Autodesk Fusion 360 part; units mm, degrees
sketch "Sketch1" plane through (0, 0, 0) normal (0, 0, 1) x (1, 0, 0)
  line L0 (0, 0) -> (28, 0)
  line L1 (28, 0) -> (28, 16)
  line L2 (28, 16) -> (0, 16)
  line L3 (0, 16) -> (0, 0)
  dimension "d1" = 28
  dimension "d2" = 16
extrude "Extrude1" add sketch "Sketch1" along normal blind 16
sketch "Sketch2" plane through (0, 0, 16) normal (0, 0, 1) x (-1, 0, 0)
  line L0 (0, -16) -> (0, 0)
  line L1 (0, 0) -> (-28, 0)
  line L2 (-28, 0) -> (-28, -16)
  line L3 (-28, -16) -> (0, -16)
  line L4 (0, -8) -> (-28, -8) construction
  line L5 (-6.5, -16) -> (-6.5, 0) construction
  line L6 (-22, -16) -> (-22, 0) construction
  circle A0 centre (-6.5, -8) radius 3.25
  circle A1 centre (-22, -8) radius 3.25
  dimension "d5" = 6.5
  dimension "d6" = 15.5
  dimension "d7" = 6.5
  dimension "d8" = 6.5
extrude "Extrude2" cut sketch "Sketch2" against normal blind 6 contours A0 | A1
sketch "Sketch3" plane through (0, 0, 0) normal (0, 0, -1) x (1, 0, 0)
  line L0 (0, 0) -> (0, -16)
  line L1 (0, -16) -> (28, -16)
  line L2 (28, -16) -> (28, 0)
  line L3 (28, 0) -> (0, 0)
  circle A0 centre (6.5, -8) radius 3.25
  circle A1 centre (22, -8) radius 3.25
extrude "Extrude3" cut sketch "Sketch3" against normal blind 6 contours A0 | A1
sketch "Sketch4" plane through (28, 0, 0) normal (1, 0, 0) x (0, 1, 0)
  line L0 (0, 0) -> (16, 0)
  line L1 (16, 0) -> (16, 16)
  line L2 (16, 16) -> (0, 16)
  line L3 (0, 16) -> (0, 0)
  line L4 (7.6128, 11.7945) -> (5.4221, 8)
  line L5 (12.2966, 8) -> (10.1058, 4.2055)
  line L6 (2.0465, 11.4373) -> (8, 14.8745)
  line L7 (5.8942, 11.7945) -> (7.6128, 11.7945)
  line L8 (3.7034, 8) -> (5.8942, 11.7945)
  line L9 (9.3314, 11.7945) -> (4.95, 4.2055)
  line L10 (13.9535, 11.4373) -> (13.9535, 4.5627)
  line L11 (6.6686, 4.2055) -> (11.05, 11.7945)
  line L12 (10.5779, 8) -> (12.2966, 8)
  line L13 (8, 14.8745) -> (13.9535, 11.4373)
  line L14 (8, 1.1255) -> (2.0465, 4.5627)
  line L15 (2.0465, 4.5627) -> (2.0465, 11.4373)
  line L16 (8.3872, 4.2055) -> (10.5779, 8)
  line L17 (5.4221, 8) -> (3.7034, 8)
  line L18 (4.95, 4.2055) -> (6.6686, 4.2055)
  line L19 (11.05, 11.7945) -> (9.3314, 11.7945)
  line L20 (10.1058, 4.2055) -> (8.3872, 4.2055)
  line L21 (13.9535, 4.5627) -> (8, 1.1255)
  line L22 (7.0257, 8) -> (8.9743, 8) construction
  line L23 (0, 8) -> (16, 8) construction
  line L24 (8, 16) -> (8, 0) construction
  point P0 (8, 8)
  point P1 (8, 8)
extrude "Extrude4" add sketch "Sketch4" along normal blind 0.4 contours L6 L10 L13 L14 L15 L21
sketch "Sketch5" plane through (0, 0, 0) normal (0, -1, 0) x (1, 0, 0)
  line L0 (0, 0) -> (28, 0)
  line L1 (28, 0) -> (28, 16)
  line L2 (28, 16) -> (0, 16)
  line L3 (0, 16) -> (0, 0)
  arc A0 (28, 9.8) -> (28, 6.2) centre (28, 8) ccw
  dimension "d25" = 1.8
sketch "Sketch6" plane through (0, 16, 0) normal (0, 1, 0) x (-1, 0, 0)
  line L0 (-28, 0) -> (0, 0)
  line L1 (0, 0) -> (0, 16)
  line L2 (0, 16) -> (-28, 16)
  line L3 (-28, 16) -> (-28, 0)
  arc A0 (-28, 6.2) -> (-28, 9.8) centre (-28, 8) ccw
extrude "Extrude8" cut sketch "Sketch5" against normal blind 2.0465 contours L1 A0
extrude "Extrude9" cut sketch "Sketch6" against normal blind 2.047 contours L3 A0
chamfer "Chamfer1" distance 0.4 angle 45 20 edges at (14, 0, 16) (28, 8, 16) (28, 0, 3.1) (28, 0, 12.9) (28, 16, 3.1) (28, 16, 12.9) (14, 16, 16) (0, 8, 16) (0, 16, 8) (14, 16, 0) (14, 0, 0) (0, 8, 0) (0, 0, 8) (28, 8, 0) (26.2, 0, 8) (28, 1.0232, 6.2) (28, 1.0232, 9.8) (26.2, 16, 8) (28, 14.9768, 6.2) (28, 14.9768, 9.8)
chamfer "Chamfer2" distance 0.4 angle 45 6 edges at (28.4, 5.0233, 13.1559) (28.4, 10.9768, 13.1559) (28.4, 2.0465, 8) (28.4, 5.0232, 2.8441) (28.4, 10.9768, 2.8441) (28.4, 13.9535, 8)
chamfer "Chamfer3" distance 0.4 angle 45 4 edges at (9.5301, 6.8247, 16) (25.0301, 6.8247, 16) (3.4699, 6.8247, 0) (18.9699, 6.8247, 0)
chamfer "Chamfer4" distance 0.6 angle 45 4 edges at (25.0301, 6.8247, 10) (9.5301, 6.8247, 10) (18.9699, 6.8247, 6) (3.4699, 6.8247, 6)
extrude "Extrude7" cut 2 faces at (7.0507, 8.6906, 10) (23.3948, 7.2286, 10) along direction (0, 0, -1) blind 4
For this review, take the finished solid that the model builds, in its own axes (mm). A direction names the side the tool comes from. Round coordinates to 2 decimals unless told otherwise and drop trailing zeros. Write each loop counter-clockwise with the first axis right and the second up, starting at its lowest first coordinate (ties: lowest second). Pieces come first, ordered by that corner, then holes. Notation, with made-up numbers: (-19, -3) -> (40, -3) arc R23 ccw to (40, 28) -> close; hole circle Ø10 at (-38.75, 34). An arc over 180 degrees is marked (long way). Put each result on its own line as item: value.
Q1. Machinability: for faces 4 (the cylindrical face through (25.247, 7.857, 13.135)), 5 (the cylindrical face through (20.777, 10.351, 8.028)), 6 (the flat face through (28, 10, 6)), which of the approach directions +Z, -Z, +X, -X, +Y, -Y give a long, thin tool a straight path to every point of the face, cutting with its end or side? Answer none if there is none.
Determined:
face 4: +Z
face 5: +Z, -Z
face 6: +X
Q2. To check wall thickness, follow L1, parallel to X at y = 8, z = 13.3; L2, parallel to X at y = 8, z = 9.15; L3, parallel to Y at x = 6, z = 13.25. State the ranges of each line that lie inside material, in increasing order. Write a range as [from, to].
Determined:
L1: x = [0, 3.25], [9.75, 18.75], [25.25, 28.4]
L2: x = [0, 3.85], [9.15, 19.35], [24.65, 28]
L3: y = [0, 4.79], [11.21, 16]
Q3. Clearance check with flat-ended pins moving along their axes: pin 1 Ø1.1 at (y, z) = (10, 5.5) entering from +X; pin 2 Ø6.5 at (y, z) = (8.5, 7.5) entering from +X; pin 3 Ø1.4 at (x, z) = (27.5, 8.5) entering from -Y; pin 4 Ø0.9 at (x, z) = (27, 8.5) entering from +Y. State where each tip first meets the part, or that it passes through.
Determined:
pin 1: stops at x = 28
pin 2: stops at x = 28.4
pin 3: stops at y = 2.05
pin 4: stops at y = 13.95
Q4. The part is to be moulded in two halves that separate along Y. For faces 1 (the flat face through (28, 7.9, 0.7)), 2 (the flat face through (28.2, 8.8, 7.9)), 3 (the flat face through (28.2, 10.92, 12.96)), say which applies: released by +Y, released by -Y, zero draft, split by the parting line, or undercut.
Determined:
face 1: zero draft
face 2: undercut
face 3: released by +Y
Q5. Consider section A-A on x = 22. State the section outline as (y, z) points, and give its area (3 significant figures).
Determined:
outline: (0, 0.4) -> (0.4, 0) -> (4.35, 0) -> (4.75, 0.4) -> (4.75, 5.4) -> (5.35, 6) -> (5.35, 10) -> (4.75, 10.6) -> (4.75, 15.6) -> (4.35, 16) -> (0.4, 16) -> (0, 15.6) -> close; (10.65, 6) -> (11.25, 5.4) -> (11.25, 0.4) -> (11.65, 0) -> (15.6, 0) -> (16, 0.4) -> (16, 15.6) -> (15.6, 16) -> (11.65, 16) -> (11.25, 15.6) -> (11.25, 10.6) -> (10.65, 10) -> close
area: 157 mm^2
Q6. Consider section B-B on z = 13. Give the number of separate pieces and of enclosed holes in the cut face, and give its area (3 significant figures).
Determined:
separate pieces: 1
enclosed holes: 2
area: 384 mm^2
